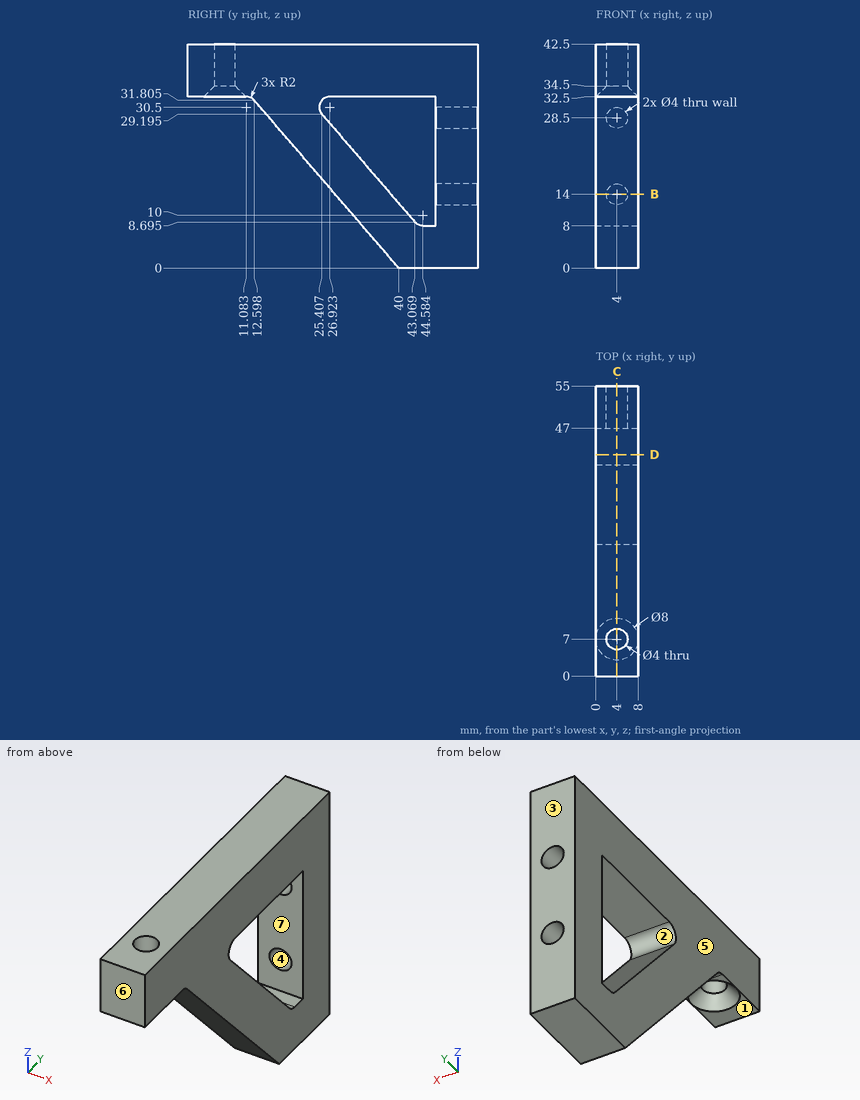
Design review of the part shown in the three views and the two pictorial views. Dimensions are in mm from the part's minimum x, y and z. A direction names the side the tool comes from. Round coordinates to 2 decimals unless told otherwise and drop trailing zeros. Loops run counter-clockwise (first coordinate to the right, second up) from the corner with the lowest first, then second, coordinate; pieces in that order, holes last. Notation, with made-up numbers: (87, -18.75) -> (131, -18.75) arc R23 cw to (131, 17.25) -> close; hole circle Ø6 at (9.25, 65). An arc over 180 degrees is marked (long way). Answer as a JSON object with one key per item and string values. Group by question number.
1) We need section B-B on z = 14. Write out the cut boundary in (x, y).
2) We need section D-D on y = 42. Write out the cut boundary in (x, z) (1 decimal).
3) For the marked faces 1, 2, 3 and 4, list the 3-axis set-ups (+Z, -Z, +X, -X, +Y, -Y) from which the entire face can be reached by the end or side of a thin tool; tool diameter is ignored.
4) Mouldability with a two-part tool opening along Y and no side actions: class the marked faces 5, 6 and 7 as released by +Y, released by -Y, zero draft, split by the parting line, or undercut.
5) We need section C-C on x = 4. Give the number of separate pieces and of enclosed holes in the cut face, then the cut area to 3 significant figures.
6) For line 1 (X direction, y = 52.25, z = 28.5); line 2 (Z direction, x = 5.25, y = 51); line 3 (Z direction, x = 7.25, y = 27) (1 decimal), list the stretches that pass through material, from the lowest coordinate up. Write a range as [from, to].
7) For pin 1 Ø4 at (x, z) = (2.5, 25.5) entering from -Y; pin 2 Ø2.5 at (x, y) = (5, 35.5) entering from -Z; pin 3 Ø3.5 at (x, z) = (4, 28.5) entering from +Y (1 decimal), all flat-tipped, find the tip position at first contact; note any pin that passes through.
Result set:
{
 "1": {"outline": "(0, 27.94) -> (8, 27.94) -> (8, 38.5) -> (0, 38.5) -> close; (0, 47) -> (2, 47) -> (2, 55) -> (0, 55) -> close; (6, 47) -> (8, 47) -> (8, 55) -> (6, 55) -> close"},
 "2": {"outline": "(0, 0) -> (8, 0) -> (8, 9.9) -> (0, 9.9) -> close; (0, 32.5) -> (8, 32.5) -> (8, 42.5) -> (0, 42.5) -> close"},
 "3": {"face 1": "-Z, +X, -X, -Y", "face 2": "+X, -X", "face 3": "+Z, -Z, +X, -X, +Y", "face 4": "+Y"},
 "4": {"face 5": "zero draft", "face 6": "released by -Y", "face 7": "undercut"},
 "5": {"separate pieces": "3", "enclosed holes": "0", "area": "1,050 mm²"},
 "6": {"line 1": "[0, 2], [6, 8]", "line 2": "[0, 12.44], [15.56, 26.94], [30.06, 42.5]", "line 3": "[15.1, 27.3], [32.5, 42.5]"},
 "7": {"pin 1": "y = 16.31", "pin 2": "z = 3.77", "pin 3": "y = 27.5"}
}
